Autodesk Inventor part; units mm, degrees
ref_plane "YZ Plane" through (0, 0, 0) normal (1, 0, 0) x (0, 1, 0)
ref_plane "XZ Plane" through (0, 0, 0) normal (0, 1, 0) x (-1, 0, 0)
ref_plane "XY Plane" through (0, 0, 0) normal (0, 0, 1) x (1, 0, 0)
sketch "Szkic1" plane through (0, 0, 0) normal (0, 0, 1) x (1, 0, 0)
  line L0 (-10.2233, 17.3341) -> (-10.2233, -75.2659)
  line L1 (-10.2233, -75.2659) -> (31.7767, -75.2659)
  line L2 (-10.2233, 17.3341) -> (31.7767, 17.3341)
  line L3 (31.7767, 17.3341) -> (31.7767, -18.9659)
  line L4 (31.7767, -75.2659) -> (31.7767, -38.9659)
  line L5 (31.7767, -38.9659) -> (51.7767, -38.9659)
  line L6 (51.7767, -38.9659) -> (51.7767, -18.9659)
  line L7 (51.7767, -18.9659) -> (31.7767, -18.9659)
  line L8 (43.2767, -28.9659) -> (40.2767, -28.9659) construction
  line L9 (43.2767, -26.9659) -> (40.2767, -26.9659)
  line L10 (40.2767, -30.9659) -> (43.2767, -30.9659)
  arc A0 (43.2767, -30.9659) -> (43.2767, -26.9659) centre (43.2767, -28.9659) ccw
  arc A1 (40.2767, -26.9659) -> (40.2767, -30.9659) centre (40.2767, -28.9659) ccw
  point P0 (0, 0)
  point P1 (-4.4733, 12.3341)
  point P2 (26.0267, 12.3341)
  point P3 (-4.4733, -13.6659)
  point P4 (26.0267, -13.6659)
  point P5 (-4.4733, -44.2659)
  point P6 (26.0267, -44.2659)
  point P7 (-4.4733, -70.2659)
  point P8 (26.0267, -70.2659)
  point P9 (41.7767, -28.9659)
  point P10 (23.2767, -28.9659)
  dimension "d0" = 92.6
  dimension "d1" = 42
  dimension "d2" = 20
  dimension "d3" = 20
  dimension "d4" = 36.3
  dimension "d39" = 5
  dimension "d40" = 5
  dimension "d41" = 5
  dimension "d42" = 5
  dimension "d43" = 5.75
  dimension "d44" = 5.75
  dimension "d45" = 42
  dimension "d46" = 5.75
  dimension "d47" = 5.75
  dimension "d48" = 5.75
  dimension "d49" = 5.75
  dimension "d50" = 36.3
  dimension "d51" = 5.75
  dimension "d52" = 5.75
  dimension "d60" = 26
  dimension "d61" = 26
  dimension "d62" = 26
  dimension "d63" = 26
  dimension "d65" = 10
  dimension "d66" = 10
  dimension "d74" = 1.5
  dimension "d75" = 4
  dimension "d76" = 33.5
  dimension "d77" = 10
extrude "Wyciągnięcie proste1" add sketch "Szkic1" along normal blind 4
chamfer "Faza1" distance 2 angle 45 2 edges at (51.7767, -18.9659, 2) (51.7767, -38.9659, 2)
hole "Otwór3" at (-4.4733, 12.3341, 0) at (26.0267, 12.3341, 0) at (-4.4733, -13.6659, 0) at (26.0267, -13.6659, 0) at (-4.4733, -44.2659, 0) at (26.0267, -44.2659, 0) at (-4.4733, -70.2659, 0) at (26.0267, -70.2659, 0) direction (0, 0, 1) diameter 5 end through all
fillet "Zaokrąglenie1" radius 1 4 edges at (31.7767, 17.3341, 2) (-10.2233, 17.3341, 2) (31.7767, -75.2659, 2) (-10.2233, -75.2659, 2)
hole "Otwór5" at (41.7767, -28.9659, 0) at (23.2767, -28.9659, 0) direction (0, 0, 1) diameter 4 end through all
equation "\"d4\" = -0.5 * d2 + 0.5 * d0"
equation "\"d45\" = d1"
properties part number "LC_ALU_4mm_X_End_Bearing_Side"
Geometry check sheet. Reference: the model listing, model coordinates, mm. A direction names the side the tool comes from. Give positions to 0.01 mm unless a question says otherwise; leave off trailing zeros. Order: outer loops, then holes, each group sorted by start corner. A loop starts at its lowest first (then second) coordinate and runs counter-clockwise, first axis right, second up. Notation, with made-up numbers: M 41.25,74.25 L 77.25,74.25 A33 ccw 77.25,107.25 Z; hole C 69.5,67.25 d3. An arc over 180 degrees is marked long. Use a Markdown table: item, result.
Item 1: Material ranges on line 1 along X through (y, z) = (-68, 1.85); line 2 along X through (y, z) = (-29.5, 1.85); line 3 along Y through (x, z) = (-6, 0.45), recorded low to high.
Answers follow:
| item | result |
|---|---|
| line 1 | x = -10.22 to -5.53, -3.42 to 24.97, 27.08 to 31.78 |
| line 2 | x = -10.22 to 21.35, 25.2 to 38.35, 45.2 to 51.78 |
| line 3 | y = -75.27 to -72.25, -68.29 to -46.25, -42.29 to -15.65, -11.69 to 10.35, 14.31 to 17.33 |
Item 2: Depth check by flat-ended pin: P1, Ø1.2, axis at y = -57.5, z = 1.5, coming from the +X side; P2, Ø4, axis at x = 26.03, y = -13.67, coming from the -Z side; P3, Ø1.5, axis at x = 41.5, z = 1, coming from the -Y side. Enter the tip coordinate at first touch or a pass-through.
Answers follow:
| item | result |
|---|---|
| P1 | stops at x = 31.78 |
| P2 | passes through |
| P3 | stops at y = -38.97 |
Item 3: Section check A-A (x = 27.5). Record the cut outline in (y, z).
Answers follow:
| item | result |
|---|---|
| outline | M -75.27,0 L -72.29,0 L -72.29,4 L -75.27,4 Z; M -68.25,0 L -46.29,0 L -46.29,4 L -68.25,4 Z; M -42.25,0 L -15.69,0 L -15.69,4 L -42.25,4 Z; M -11.65,0 L 10.31,0 L 10.31,4 L -11.65,4 Z; M 14.35,0 L 17.33,0 L 17.33,4 L 14.35,4 Z |
Item 4: Section check C-C (z = 2.45). State how many separate pieces and enclosed holes the cut face has, and give its area (3 significant figures).
Answers follow:
| item | result |
|---|---|
| separate pieces | 1 |
| enclosed holes | 10 |
| area | 4,090 mm2 |
Item 5: Tool access check on faces 1 (the flat face through (31.777, -1, 2)), 2 (the flat face through (50.76, -37.98, 1.97)), 3 (the cylindrical face through (45.276, -28.922, 1.972)). Record the directions out of +Z, -Z, +X, -X, +Y, -Y that give a thin tool (end or side, any length) a straight path to the whole face; none if there is none.
Answers follow:
| item | result |
|---|---|
| face 1 | +Z, -Z, +X, +Y |
| face 2 | +Z, -Z, +X, -Y |
| face 3 | +Z, -Z |
Item 6: Section check D-D (y = -63). Record the cut outline in (x, z).
Answers follow:
| item | result |
|---|---|
| outline | M -10.22,0 L 31.78,0 L 31.78,4 L -10.22,4 Z |
Item 7: Section check B-B (y = -14.5). Record the cut outline in (x, z).
Answers follow:
| item | result |
|---|---|
| outline | M -10.22,0 L -6.83,0 L -6.83,4 L -10.22,4 Z; M -2.12,0 L 23.67,0 L 23.67,4 L -2.12,4 Z; M 28.38,0 L 31.78,0 L 31.78,4 L 28.38,4 Z |
